Geometry: final body of the model. Coordinates: model frame, mm. Give positions to 0.01 mm unless a question says otherwise; leave off trailing zeros. Write each loop counter-clockwise with the first axis right and the second up, starting at its lowest first coordinate (ties: lowest second). Pieces come first, ordered by that corner, then holes. Notation, with made-up numbers: (39.5, 88) -> (98.5, 88) arc R24 ccw to (98.5, 111) -> close; hole circle Ø7 at (82, 80.5). An arc over 180 degrees is marked (long way). Answer as a JSON object with one key per item and string values. Group by question number.
(1) Section query C-C on x = -30. Output: boundary loops of the cut face in (y, z), plus the area to 3 significant figures.
(2) Section query A-A on y = -16.5. Output: boundary loops of the cut face in (x, z), plus the area to 3 significant figures.
(3) Contact query for flat-ended pins moving along their axis: pin 1 Ø4.5 at (x, y) = (-34.64, 22.9) entering from -Z; pin 2 Ø3.5 at (x, y) = (20.36, 14.76) entering from +Z. Output: stop coordinate, or through.
(4) Section query D-D on x = 12. Output: boundary loops of the cut face in (y, z), plus the area to 3 significant figures.
(5) Section query B-B on z = 2.05. Output: boundary loops of the cut face in (x, y), plus the area to 3 significant figures.
(6) Material intervals for probe 1 along X at (y, z) = (14.5, 2.45) (3 decimals); probe 2 along Y at (x, z) = (21, 1.1); probe 3 along Y at (x, z) = (-26, 1.9), sorted ascending.
from build123d import *

# Parameters (mm, degrees)
SKETCH_1_R      = 2
EXTRUDE_1_DEPTH = 3


with BuildPart() as part:
    # 草图1 → 凸台-拉伸1 (new body)
    with BuildSketch(Plane.XY):
        with BuildLine():
            Line((-8.253871793, -13.107166096), (22.860072418, -31.070810161))
            ThreePointArc((22.860072418, -31.070810161), (27.860072418, -31.070810161), (30.360072418, -26.740683142))
            Line((30.360072418, -26.740683142), (30.360072418, 24.757413889))
            Line((30.360072418, 24.757413889), (10.360072418, 24.757413889))
            Line((10.360072418, 24.757413889), (10.360072418, 7.900333009))
            ThreePointArc((10.360072418, 7.900333009), (7.860072418, 3.57020599), (2.860072418, 3.57020599))
            Line((2.860072418, 3.57020599), (-8.514722631, 10.137446974))
            ThreePointArc((-8.514722631, 10.137446974), (-20.277530658, 21.869741204), (-24.639927582, 37.900333009))
            Line((-24.639927582, 37.900333009), (-44.639927582, 37.900333009))
            Line((-44.639927582, 37.900333009), (-44.639927582, -22.099666991))
            Line((-44.639927582, -22.099666991), (-24.639927582, -22.099666991))
            ThreePointArc((-24.639927582, -22.099666991), (-18.978211718, -12.990882096), (-8.253871793, -13.107166096))
        make_face()
        with Locations((-34.639927582, 22.900333009)):
            Circle(SKETCH_1_R, mode=Mode.SUBTRACT)
        with Locations((-34.639927582, 7.900333009)):
            Circle(SKETCH_1_R, mode=Mode.SUBTRACT)
        with Locations((-34.639927582, -7.099666991)):
            Circle(SKETCH_1_R, mode=Mode.SUBTRACT)
        with Locations((-11.649546525, 0.400333009)):
            Circle(SKETCH_1_R, mode=Mode.SUBTRACT)
        with Locations((1.340834531, -7.099666991)):
            Circle(SKETCH_1_R, mode=Mode.SUBTRACT)
        with Locations((20.360072418, 4.757413889)):
            Circle(SKETCH_1_R, mode=Mode.SUBTRACT)
        with Locations((20.360072418, 14.757413889)):
            Circle(SKETCH_1_R, mode=Mode.SUBTRACT)
    extrude(amount=EXTRUDE_1_DEPTH)


solid = part.part
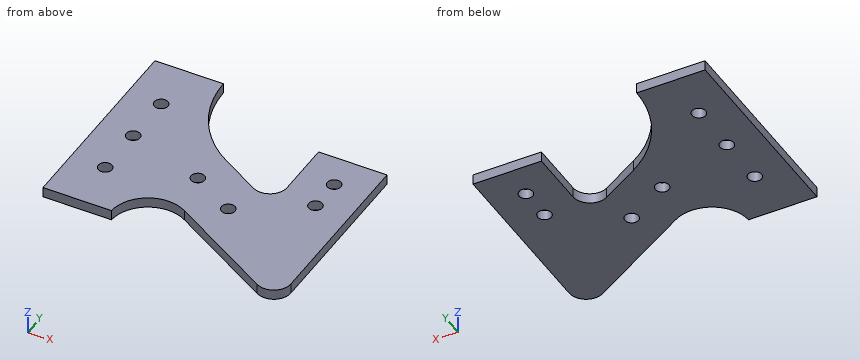
Answer list:
{
 "1": {"outline": "(-22.1, 0) -> (37.9, 0) -> (37.9, 3) -> (-22.1, 3) -> close", "area": "180 mm2"},
 "2": {"outline": "(-44.64, 0) -> (-22.81, 0) -> (-22.81, 3) -> (-44.64, 3) -> close; (-2.38, 0) -> (30.36, 0) -> (30.36, 3) -> (-2.38, 3) -> close", "area": "164 mm2"},
 "3": {"pin 1": "z = 0", "pin 2": "through"},
 "4": {"outline": "(-24.8, 0) -> (24.76, 0) -> (24.76, 3) -> (-24.8, 3) -> close", "area": "149 mm2"},
 "5": {"outline": "(-44.64, -22.1) -> (-24.64, -22.1) arc R10.93 cw to (-8.25, -13.11) -> (22.86, -31.07) arc R5 ccw to (30.36, -26.74) -> (30.36, 24.76) -> (10.36, 24.76) -> (10.36, 7.9) arc R5 cw to (2.86, 3.57) -> (-8.51, 10.14) arc R32.25 cw to (-24.64, 37.9) -> (-44.64, 37.9) -> close; hole circle Ø4 at (-34.64, -7.1); hole circle Ø4 at (-34.64, 7.9); hole circle Ø4 at (-34.64, 22.9); hole circle Ø4 at (-11.65, 0.4); hole circle Ø4 at (1.34, -7.1); hole circle Ø4 at (20.36, 4.76); hole circle Ø4 at (20.36, 14.76)", "area": "3,150 mm2"},
 "6": {"probe 1": "-44.64 to -14.405, 10.36 to 18.377, 22.343 to 30.36", "probe 2": "-30 to 2.86, 6.65 to 12.86, 16.65 to 24.76", "probe 3": "-22.1 to 37.9"}
}
